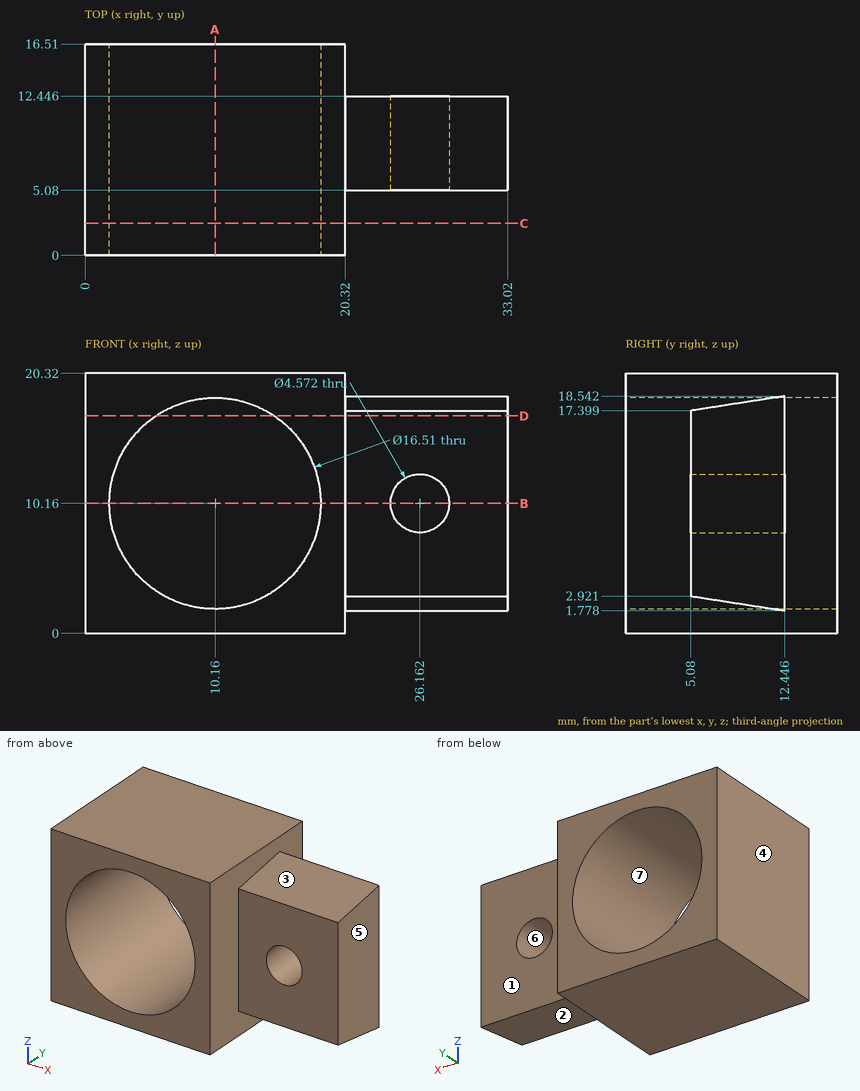
Drawing for the job (mm, zero at the part's lowest x, y, z). A direction names the side the tool comes from. Round coordinates to 2 decimals unless told otherwise and drop trailing zeros. Write each loop counter-clockwise with the first axis right and the second up, starting at its lowest first coordinate (ties: lowest second). Pieces come first, ordered by that corner, then holes. Notation, with made-up numbers: M 30.5,51 L 81.5,51 A33 ccw 81.5,88 Z; hole C 59,26.25 d7. An arc over 180 degrees is marked long. Answer as a JSON object with one key per item and string values. Group by question number.
(1) Drill centre lines: L1, parallel to Z at x = 10, y = 5; L2, parallel to Y at x = 25.5, z = 14.25; L3, parallel to X at y = 12, z = 11.75. Where is each one in solid material? Low to high.
(2) Flat gauge pins, fed straight in: pin 1 (6 mm diameter, centred on x = 26.162, z = 10.16, fed in from -Y); pin 2 (8 mm diameter, centred on y = 15, z = 2.5, fed in from +X); pin 3 (1 mm diameter, centred on x = 26, y = 7, fed in from +Z); pin 4 (10 mm diameter, centred on x = 25.5, z = 11, fed in from +Y). Where does each tip first touch, or does it go through?
(3) Cut at C-C (y = 2.5). Give the cut face in (x, z) (3 decimals), and give its area (3 significant figures).
(4) Cut at D-D (z = 17). Give the cut face in (x, y).
(5) Mould opens along X. For the marked faces 4, 5, 6 and 7 say: pulls with the +X half, pulls with the -X half, needs draft (parallel to the pull), parting line crosses it, or undercut.
(6) Which spindle directions (+Z, -Z, +X, -X, +Y, -Y) get a long thin tool onto all of the face, cutting with end or side? Do the marked faces 1, 2 and 3. Say none if no direction does.
(7) Cut at B-B (z = 10.16). Give the cut face in (x, y) (3 decimals), and give its area (3 significant figures).
(8) Cut at A-A (x = 10.16). Give the cut face in (y, z) (3 decimals), and give its area (3 significant figures).
Responses:
{
 "1": {"L1": "z = 0 to 1.91, 18.41 to 20.32", "L2": "y = 5.08 to 12.45", "L3": "x = 0 to 2.06, 18.26 to 24.52, 27.8 to 33.02"},
 "2": {"pin 1": "stops at y = 5.08", "pin 2": "stops at x = 33.02", "pin 3": "stops at z = 17.77", "pin 4": "stops at y = 12.45"},
 "3": {"outline": "M 0,0 L 20.32,0 L 20.32,20.32 L 0,20.32 Z; hole C 10.16,10.16 d16.51", "area": "199 mm2"},
 "4": {"outline": "M 0,0 L 5.54,0 L 5.54,16.51 L 0,16.51 Z; M 14.78,0 L 20.32,0 L 20.32,5.08 L 33.02,5.08 L 33.02,12.45 L 20.32,12.45 L 20.32,16.51 L 14.78,16.51 Z"},
 "5": {"face 4": "pulls with the -X half", "face 5": "pulls with the +X half", "face 6": "undercut", "face 7": "undercut"},
 "6": {"face 1": "+Z, -Z, +X, +Y", "face 2": "-Z, +X, -Y", "face 3": "+Z, +X, -Y"},
 "7": {"outline": "M 0,0 L 1.905,0 L 1.905,16.51 L 0,16.51 Z; M 18.415,0 L 20.32,0 L 20.32,5.08 L 23.876,5.08 L 23.876,12.446 L 20.32,12.446 L 20.32,16.51 L 18.415,16.51 Z; M 28.448,5.08 L 33.02,5.08 L 33.02,12.446 L 28.448,12.446 Z", "area": "123 mm2"},
 "8": {"outline": "M 0,0 L 16.51,0 L 16.51,1.905 L 0,1.905 Z; M 0,18.415 L 16.51,18.415 L 16.51,20.32 L 0,20.32 Z", "area": "62.9 mm2"}
}
